Source: CAD feature listing. Evaluate the final solid. Frame: model axes, mm. Round coordinates to 2 decimals unless told otherwise and drop trailing zeros. Loops run counter-clockwise (first coordinate to the right, second up) from the corner with the lowest first, then second, coordinate; pieces in that order, holes last.
Item 1: Section query A-A on y = 61. Return loops of the section in (x, z).
Item 2: First-contact query: P1, Ø1, axis at x = -2.5, y = 391, coming from the +Z side; P2, Ø3, axis at x = -2, z = 854.5, coming from the +Y side. Flat tips, straight axial feed; report the tip coordinate or a pass-through.
Item 3: Section query B-B on x = -5. Give the number of separate pieces and of enclosed holes in the cut face, then the cut area to 3 significant figures.
Item 4: Ray query, L1, parallel to Y at x = -2, z = 817; L2, parallel to Z at x = -4.5, y = 317; L3, parallel to Z at x = -1, y = 260. Return the intervals inside material, ascending.
Item 5: Section query C-C on z = 515.5. Return loops of the section in (x, y), then the cut area to 3 significant figures.
```python
from build123d import *

# Parameters (mm, degrees)
BASE_FLANGE1_DEPTH               = 6.35
F_1_4_CLEARANCE_HOLE1_D          = 6.7564
CUT_EXTRUDE1_DEPTH               = 1200.074385724
F_27_32_0_84375_DIAMETER_HOLE1_D = 21.43125
CUT_EXTRUDE2_DEPTH               = 1200.074385724
CUT_EXTRUDE3_DEPTH               = 1200.074385724
CUT_EXTRUDE5_DEPTH               = 1200.074385724
CUT_EXTRUDE6_DEPTH               = 1183.362497291
CUT_EXTRUDE7_DEPTH               = 1183.362497291
CUT_EXTRUDE8_DEPTH               = 1183.362497291
F_5_8_0_625_DIAMETER_HOLE1_D     = 15.875
FILLET2_R                        = 3.556


# Sheet-metal steps are written as plain solids
with BuildPart() as part:
    # Sketch1 → Base-Flange1 (new body)
    with BuildSketch(Plane(origin=(0, 0, 0), x_dir=(0, 0, -1), z_dir=(1, 0, 0))):
        with BuildLine():
            Line((-1054.1, 247.773526455), (-876.3, 520.7))
            Line((-876.3, 520.7), (-800.1, 520.7))
            Line((-800.1, 520.7), (-800.1, 571.5))
            Line((-800.1, 571.5), (-438.15, 571.5))
            Line((-438.15, 571.5), (-438.15, 125.253453767))
            Line((-438.15, 125.253453767), (-438.15, 0))
            Line((-438.15, 0), (-790.575, 0))
            ThreePointArc((-790.575, 0), (-844.607803402, 151.01156908), (-982.176450511, 233.467042956))
            Line((-982.176450511, 233.467042956), (-1054.1, 247.773526455))
        make_face()
    extrude(amount=-BASE_FLANGE1_DEPTH)

    # 1/4 Clearance Hole1 (through all)
    with Locations(Plane(origin=(0, 0, 0), x_dir=(0, 0, -1), z_dir=(1, 0, 0))):
        with Locations((-704.85, 22.225), (-1011.776786637, 265.252531308), (-488.62591807, 161.191353545), (-875.60064198, 445.346335342), (-526.833396269, 375.972216833), (-850.688695858, 440.391041163), (-744.812924838, 419.331040901), (-890.331049291, 241.095472185), (-784.455278272, 220.035471923), (-619.125, 549.275)):
            Hole(F_1_4_CLEARANCE_HOLE1_D / 2)

    # Sketch11 → Cut-Extrude1 (cut, through all)
    with BuildSketch(Plane(origin=(0, 0, 0), x_dir=(0, 0, -1), z_dir=(1, 0, 0))):
        Polygon((-845.296687768, 345.439648176), (-786.130815728, 333.670824501), (-792.324933452, 302.530891848), (-851.490805492, 314.299715524), align=None)
    extrude(amount=-CUT_EXTRUDE1_DEPTH, mode=Mode.SUBTRACT)

    # 27/32 (0.84375) Diameter Hole1 (through all)
    with Locations(Plane(origin=(0, 0, 0), x_dir=(0, 0, -1), z_dir=(1, 0, 0))):
        with Locations((-849.855910604, 239.518870383), (-822.45276987, 234.068046786)):
            Hole(F_27_32_0_84375_DIAMETER_HOLE1_D / 2)

    # Sketch14 → Cut-Extrude2 (cut, through all)
    with BuildSketch(Plane(origin=(0, 0, 0), x_dir=(0, 0, -1), z_dir=(1, 0, 0))):
        Polygon((-864.197214028, 258.557542635), (-870.391331752, 227.417609982), (-808.111466446, 215.029374534), (-801.917348722, 246.169307187), (-794.484407453, 283.53722637), (-856.764272759, 295.925461818), align=None)
    extrude(amount=-CUT_EXTRUDE2_DEPTH, mode=Mode.SUBTRACT)

    # Sketch15 → Cut-Extrude3 (cut, through all)
    with BuildSketch(Plane(origin=(0, 0, 0), x_dir=(0, 0, -1), z_dir=(1, 0, 0))):
        Polygon((-438.15, 571.5), (-476.25, 571.5), (-476.25, 523.875), (-438.15, 501.877954744), align=None)
        Polygon((-438.15, 0), (-495.3, 0), (-495.3, 50.8), (-438.15, 88.9), align=None)
    extrude(amount=-CUT_EXTRUDE3_DEPTH, mode=Mode.SUBTRACT)

    # Sketch17 → Cut-Extrude5 (cut, through all)
    with BuildSketch(Plane.ZY.offset(6.35)):
        Polygon((1035.05, 277.01564862), (1035.05, 243.984245856), (1054.1, 247.773526455), align=None)
    extrude(amount=-CUT_EXTRUDE5_DEPTH, mode=Mode.SUBTRACT)

    # Sketch18 → Cut-Extrude6 (cut, through all)
    with BuildSketch(Plane.ZY.offset(6.35)):
        Polygon((476.25, 523.875), (438.15, 501.877954744), (438.15, 470.127954744), (527.05, 523.875), (527.05, 571.5), (476.25, 571.5), align=None)
    extrude(amount=-CUT_EXTRUDE6_DEPTH, mode=Mode.SUBTRACT)

    # Sketch20 → Cut-Extrude7 (cut, through all)
    with BuildSketch(Plane.ZY.offset(6.35)):
        with BuildLine():
            Line((438.15, 298.599947238), (438.15, 222.399947238))
            ThreePointArc((438.15, 222.399947238), (463.55, 260.499947238), (438.15, 298.599947238))
        make_face()
    extrude(amount=-CUT_EXTRUDE7_DEPTH, mode=Mode.SUBTRACT)

    # Sketch22 → Cut-Extrude8 (cut, through all)
    with BuildSketch(Plane.ZY.offset(6.35)):
        Polygon((800.1, 520.7), (762, 571.5), (800.1, 571.5), align=None)
    extrude(amount=-CUT_EXTRUDE8_DEPTH, mode=Mode.SUBTRACT)

    # 5/8 (0.625) Diameter Hole1 (through all)
    with Locations(Plane(origin=(0, 0, 0), x_dir=(0, 0, -1), z_dir=(1, 0, 0))):
        with Locations((-823.332971453, 480.270476242), (-754.825119616, 466.643417249), (-817.385708629, 152.130097456), (-829.173016653, 361.400764358), (-794.919090735, 354.587234862)):
            Hole(F_5_8_0_625_DIAMETER_HOLE1_D / 2)

    # Fillet2
    fillet2_edges = [part.edges().sort_by_distance(p)[0] for p in [
        (-3.175, 314.299715524, 851.490805492),
        (-3.175, 345.439648176, 845.296687768),
        (-3.175, 333.670824501, 786.130815728),
        (-3.175, 302.530891848, 792.324933452),
        (-3.175, 295.925461818, 856.764272759),
        (-3.175, 283.53722637, 794.484407453),
        (-3.175, 215.029374534, 808.111466446),
        (-3.175, 227.417609982, 870.391331752),
        (-3.175, 520.7, 800.1),
        (-3.175, 50.8, 495.3),
        (-3.175, 277.01564862, 1035.05),
        (-3.175, 243.984245856, 1035.05),
        (-3.175, 523.875, 527.05),
    ]]
    fillet(fillet2_edges, radius=FILLET2_R)


solid = part.part
```
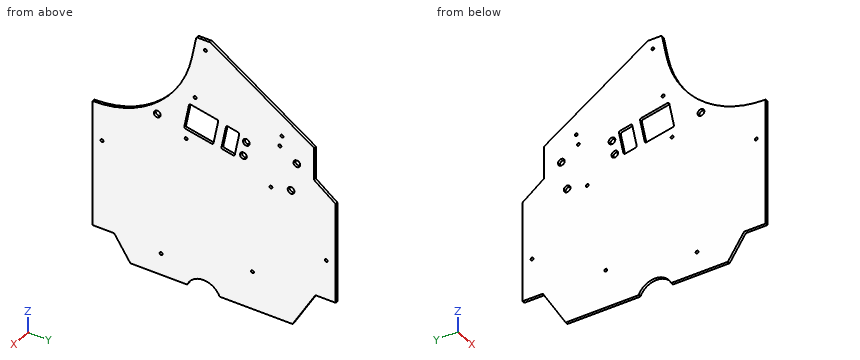
Data:
1. outline: (-6.35, 480) - (0, 480) - (0, 798.52) - (-6.35, 798.52) - close
2. P1: stops at z = 961.12
2. P2: stops at y = 520.7
3. separate pieces: 1
3. enclosed holes: 17
3. area: 243,000 mm2
4. L1: y = 109.01 to 144.2, 160.06 to 216.8, 288.02 to 307.44, 339.81 to 475.49, 485.06 to 520.7
4. L2: z = 438.15 to 789.45, 850.86 to 1009
4. L3: z = 463.55 to 799.17, 863.91 to 1035.05
5. outline: (-6.35, 0) - (0, 0) - (0, 516.89) - (-6.35, 516.89) - close
5. area: 3,280 mm2
